from build123d import *

# Parameters (mm, degrees)
F0_W     = 101.6
F0_H     = 44.45
F1_DEPTH = 21.59
F2_T     = -1.5
F4_DEPTH = 1.5


# Not quite as in the source:
# - a pattern or mirror of a feature is missing from the dataset's text; its kind, count and spacing are read off the source's solid


with BuildPart() as f1:
    # F0 (on Top) → F1 (new body)
    with BuildSketch(Plane.XY):
        Rectangle(F0_W, F0_H)
    extrude(amount=F1_DEPTH)

    # F2
    f2_openings = [f1.faces().sort_by_distance(p)[0] for p in [
        (0, 0, 21.59),
    ]]
    offset(amount=F2_T, openings=f2_openings)

    # F3 (on face) → F4 (cut)
    with BuildSketch(Plane(origin=(-50.8, 0, 0), x_dir=(0, -1, 0), z_dir=(-1, 0, 0))):
        with BuildLine():
            ThreePointArc((-14.5911212754, 15.4684429111), (0.3183541842, 1.5034700934), (14.605, 16.105))
            ThreePointArc((14.605, 16.105), (14.6032460444, 16.3313403807), (14.5979845987, 16.5576263976))
            ThreePointArc((14.5979845987, 16.5576263976), (14.290212434, 19.1209332868), (13.5359078011, 21.59))
            Line((13.5359078011, 21.59), (-13.5359078011, 21.59))
            ThreePointArc((-13.5359078011, 21.59), (-14.2709246664, 19.2109192145), (-14.5911212754, 16.7415570889))
            Line((-14.5911212754, 16.7415570889), (-14.5911212754, 15.4684429111))
        make_face()
        with BuildLine():
            ThreePointArc((13.5359078011, 21.59), (14.290212434, 19.1209332868), (14.5979845987, 16.5576263976))
            Line((14.5979845987, 16.5576263976), (14.5979845987, 21.59))
            Line((14.5979845987, 21.59), (13.5359078011, 21.59))
        make_face()
        with BuildLine():
            Line((-14.5911212754, 21.59), (-14.5911212754, 16.7415570889))
            ThreePointArc((-14.5911212754, 16.7415570889), (-14.2709246664, 19.2109192145), (-13.5359078011, 21.59))
            Line((-13.5359078011, 21.59), (-14.5911212754, 21.59))
        make_face()
    f4 = extrude(amount=-F4_DEPTH, mode=Mode.SUBTRACT)

    # F4_copies: F4 across plane
    add(f4.mirror(Plane(origin=(0, 0, 0), x_dir=(0, 0, 1), z_dir=(1, 0, 0))), mode=Mode.SUBTRACT)


solid = f1.part
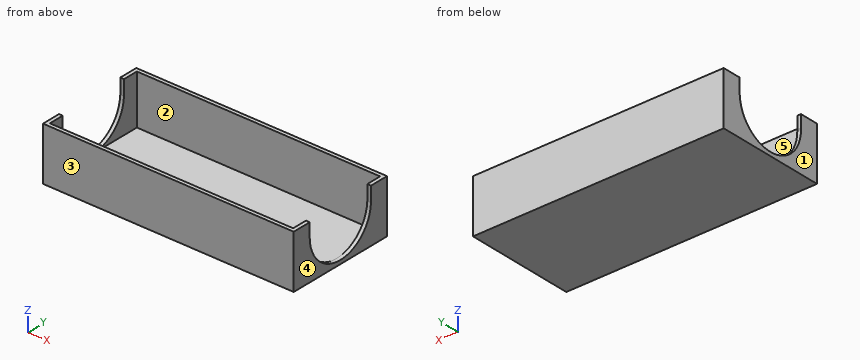
Part model, mm, in its own coordinate system. Face numbers are marked on the shaded views. A direction names the side the tool comes from. Round coordinates to 2 decimals unless told otherwise and drop trailing zeros. Order: outer loops, then holes, each group sorted by start corner. A loop starts at its lowest first (then second) coordinate and runs counter-clockwise, first axis right, second up. Notation, with made-up numbers: (-15, 50) -> (14, 50) arc R29 ccw to (14, 86) -> close; hole circle Ø4 at (49.25, 65.5). An arc over 180 degrees is marked (long way). Put each result on its own line as item: value.
Q1. Wall check: line 1 (X direction, y = 19, z = 17); line 2 (Y direction, x = 13.5, z = 4.5) (3 decimals); line 3 (Z direction, x = 3, y = 1.5). Give the ranges that are in metal, low to high. Write a range as [from, to].
From the geometry:
line 1: x = [-50.8, -49.3], [49.3, 50.8]
line 2: y = [-22.225, -20.725], [20.725, 22.225]
line 3: z = [0, 1.5]
Q2. Band-saw the part on C-C (y = -10). Give the cut face in (x, z).
From the geometry:
outline: (-50.8, 0) -> (50.8, 0) -> (50.8, 5.46) -> (49.3, 5.46) -> (49.3, 1.5) -> (-49.3, 1.5) -> (-49.3, 5.46) -> (-50.8, 5.46) -> close
Q3. Band-saw the part on D-D (z = 5.5). Give the cut face in (x, y) (3 decimals).
From the geometry:
outline: (-50.8, -22.225) -> (50.8, -22.225) -> (50.8, -10.042) -> (49.3, -10.042) -> (49.3, -20.725) -> (-49.3, -20.725) -> (-49.3, -10.042) -> (-50.8, -10.042) -> close; (-50.8, 10.042) -> (-49.3, 10.042) -> (-49.3, 20.725) -> (49.3, 20.725) -> (49.3, 10.042) -> (50.8, 10.042) -> (50.8, 22.225) -> (-50.8, 22.225) -> close
Q4. Band-saw the part on B-B (x = 3). Give the cut face in (y, z) (3 decimals).
From the geometry:
outline: (-22.225, 0) -> (22.225, 0) -> (22.225, 21.59) -> (20.725, 21.59) -> (20.725, 1.5) -> (-20.725, 1.5) -> (-20.725, 21.59) -> (-22.225, 21.59) -> close
Q5. Pin check, flat tip, straight feed: pin 1 Ø20.5 at (x, y) = (0, 1.5) entering from +Z. Stop position of the tip, or through.
From the geometry:
pin 1: stops at z = 1.5
Q6. Band-saw the part on A-A (z = 20.25). Give the cut face in (x, y) (3 decimals), and give its area (3 significant figures).
From the geometry:
outline: (-50.8, -22.225) -> (50.8, -22.225) -> (50.8, -14.598) -> (49.3, -14.598) -> (49.3, -20.725) -> (-49.3, -20.725) -> (-49.3, -14.598) -> (-50.8, -14.598) -> close; (-50.8, 14.591) -> (-49.3, 14.591) -> (-49.3, 20.725) -> (49.3, 20.725) -> (49.3, 14.591) -> (50.8, 14.591) -> (50.8, 22.225) -> (-50.8, 22.225) -> close
area: 342 mm2
Q7. Tool access for the marked faces 1 and 2: list every direction of +Z, -Z, +X, -X, +Y, -Y with a clear straight run to the whole face (end or side of a thin tool).
From the geometry:
face 1: +Z, -Z, -X, +Y, -Y
face 2: +Z
Q8. Pull direction Y, two halves, no side cores. Call the marked faces 3, 4 and 5: pulls with the +Y half, pulls with the -Y half, needs draft (parallel to the pull), parting line crosses it, or undercut.
From the geometry:
face 3: pulls with the -Y half
face 4: needs draft
face 5: undercut
